Read the model definition and answer for the solid it produces. Units are mm, in the model's axes. Coordinates: 2 decimals unless noted, no trailing zeros. Loops run counter-clockwise (first coordinate to the right, second up) from the corner with the lowest first, then second, coordinate; pieces in that order, holes last. Notation, with made-up numbers: (77, -10.75) -> (109, -10.75) arc R34 cw to (109, 24.25) -> close; hole circle Ø5 at (51.25, 67). An arc over 180 degrees is marked (long way). Answer as CSV lines item,"result".
```python
from build123d import *

# Parameters (mm, degrees)
F1_DEPTH = 1.3208
F2_R     = 3.175
F3_DEPTH = 25.4
F4_R     = 12.7


with BuildPart() as f1:
    # F0 (on Front) → F1 (new body)
    with BuildSketch(Plane.XZ):
        Polygon((0, 2260.6), (0, 0), (1244.6, 0), (1244.6, 1955.8), align=None)
    extrude(amount=F1_DEPTH)

    # F2 (on face) → F3 (cut)
    with BuildSketch(Plane.XZ.offset(1.3208)):
        with Locations((25.4, 2228.229)):
            Circle(F2_R)
        with Locations((1219.2, 1935.869816)):
            Circle(F2_R)
        with Locations((410.443912, 2133.932531)):
            Circle(F2_R)
        with Locations((843.355338, 2027.913407)):
            Circle(F2_R)
        with Locations((1219.2, 25.4)):
            Circle(F2_R)
        with Locations((25.4, 25.4)):
            Circle(F2_R)
        with Locations((421.263099, 25.4)):
            Circle(F2_R)
        with Locations((794.35122, 25.4)):
            Circle(F2_R)
        with Locations((1219.2, 980.634908)):
            Circle(F2_R)
        with Locations((1219.2, 1489.178419)):
            Circle(F2_R)
        with Locations((1219.2, 513.280332)):
            Circle(F2_R)
        with Locations((25.4, 1346.962094)):
            Circle(F2_R)
        with Locations((25.4, 890.889168)):
            Circle(F2_R)
        with Locations((25.4, 498.568296)):
            Circle(F2_R)
        with Locations((25.4, 1842.267275)):
            Circle(F2_R)
    extrude(amount=-F3_DEPTH, mode=Mode.SUBTRACT)

    # F4
    f4_edges = [f1.edges().sort_by_distance(p)[0] for p in [
        (1244.6, -0.6604, 1955.8),
        (0, -0.6604, 2260.6),
        (1244.6, -0.6604, 0),
        (0, -0.6604, 0),
    ]]
    fillet(f4_edges, radius=F4_R)


solid = f1.part
```
Q1. Find the intervals of material crossed by probe 1 along Z at (x, y) = (1219.2, -0.5) (3 decimals); probe 2 along Z at (x, y) = (50, -0.85); probe 3 along Z at (x, y) = (935.5, -0.55), in increasing order. Write a range as [from, to].
Results:
probe 1,"z = [0, 22.225], [28.575, 510.105], [516.455, 977.46], [983.81, 1486.003], [1492.353, 1932.695], [1939.045, 1962.02]"
probe 2,"z = [0, 2248.36]"
probe 3,"z = [0, 2031.5]"
Q2. A cutting plane is placed at B-B, the plane x = 1147. Write down the section's boundary in (y, z).
Results:
outline,"(-1.32, 0) -> (0, 0) -> (0, 1979.7) -> (-1.32, 1979.7) -> close"
Q3. A cutting plane is placed at A-A, the plane y = -0.25. Give the number of separate pieces and of enclosed holes in the cut face, and give its area (3 significant figures).
Results:
separate pieces,"1"
enclosed holes,"15"
area,"2,620,000 mm²"
Q4. A cutting plane is placed at C-C, the plane x = 326. Write down the section's boundary in (y, z).
Results:
outline,"(-1.32, 0) -> (0, 0) -> (0, 2180.76) -> (-1.32, 2180.76) -> close"
